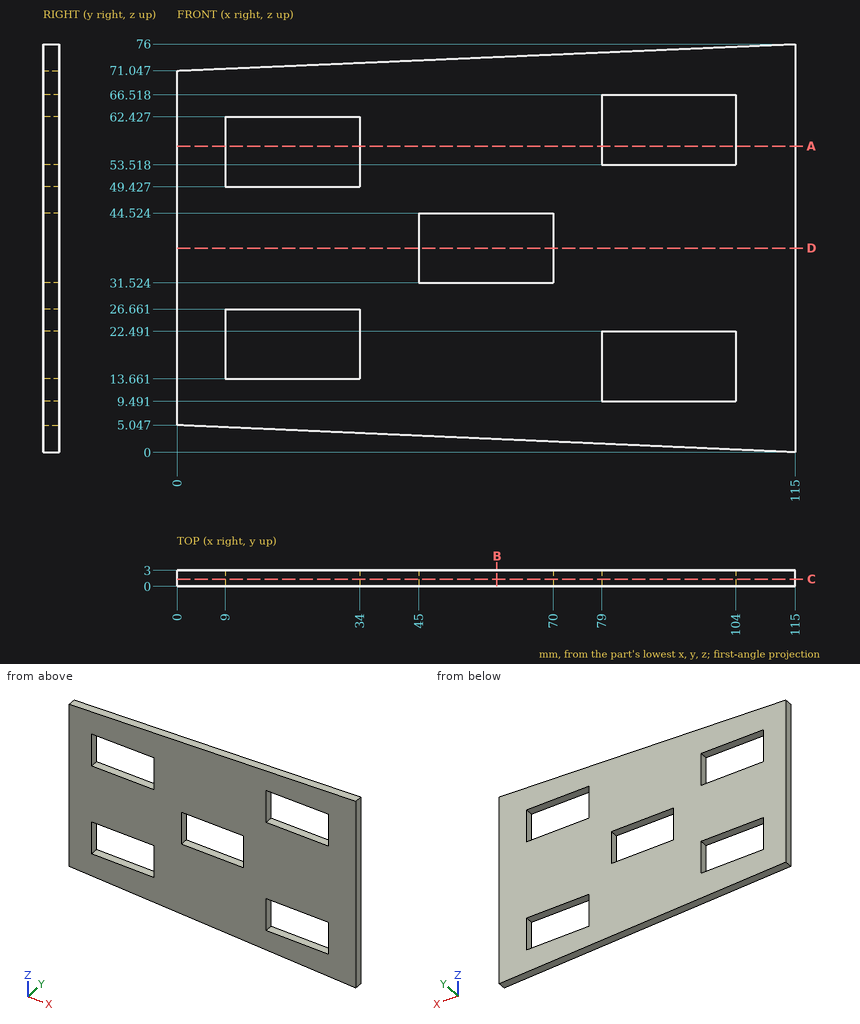
Design review of the part shown in the three views and the two pictorial views. Dimensions are in mm from the part's minimum x, y and z. Round coordinates to 2 decimals unless told otherwise and drop trailing zeros. Loops run counter-clockwise (first coordinate to the right, second up) from the corner with the lowest first, then second, coordinate; pieces in that order, holes last. Notation, with made-up numbers: (8, -11) -> (32, -11) arc R15 ccw to (32, 16) -> close; hole circle Ø4 at (-35.5, 51.25). An arc over 180 degrees is marked (long way). Return JSON: item names as keys, results as strings.
(1) Add section C-C on y = 1.35. Write out the cut boundary in (x, z), plus the area to 3 significant figures.
Solved:
{"outline": "(0, 5.05) -> (115, 0) -> (115, 76) -> (0, 71.05) -> close; hole (9, 13.66) -> (34, 13.66) -> (34, 26.66) -> (9, 26.66) -> close; hole (9, 49.43) -> (34, 49.43) -> (34, 62.43) -> (9, 62.43) -> close; hole (45, 31.52) -> (70, 31.52) -> (70, 44.52) -> (45, 44.52) -> close; hole (79, 9.49) -> (104, 9.49) -> (104, 22.49) -> (79, 22.49) -> close; hole (79, 53.52) -> (104, 53.52) -> (104, 66.52) -> (79, 66.52) -> close", "area": "6,540 mm2"}
(2) For pin 1 (0.9 mm diameter, centred on x = 18.5, y = 1, fed in from -Z); pin 2 (1 mm diameter, centred on x = 69.5, y = 0.5, fed in from +Z); pin 3 (0.9 mm diameter, centred on x = 63.5, y = 1.5, fed in from +Z), all flat-tipped, find the tip position at first contact; note any pin that passes through.
Solved:
{"pin 1": "z = 4.22", "pin 2": "z = 74.06", "pin 3": "z = 73.8"}
(3) Add section A-A on z = 57. Write out the cut boundary in (x, y), plus the area to 3 significant figures.
Solved:
{"outline": "(0, 0) -> (9, 0) -> (9, 3) -> (0, 3) -> close; (34, 0) -> (79, 0) -> (79, 3) -> (34, 3) -> close; (104, 0) -> (115, 0) -> (115, 3) -> (104, 3) -> close", "area": "195 mm2"}
(4) For line 1 (X direction, y = 2.6, z = 59); line 2 (X direction, y = 1.5, z = 33); line 3 (Z direction, x = 101, y = 1.55) (1 decimal), list the stretches that pass through material, from the lowest coordinate up.
Solved:
{"line 1": "0 to 9, 34 to 79, 104 to 115", "line 2": "0 to 45, 70 to 115", "line 3": "0.6 to 9.5, 22.5 to 53.5, 66.5 to 75.4"}
(5) Add section D-D on z = 38. Write out the cut boundary in (x, y), plus the area to 3 significant figures.
Solved:
{"outline": "(0, 0) -> (45, 0) -> (45, 3) -> (0, 3) -> close; (70, 0) -> (115, 0) -> (115, 3) -> (70, 3) -> close", "area": "270 mm2"}
(6) Add section B-B on x = 59.5. Write out the cut boundary in (y, z) (1 decimal).
Solved:
{"outline": "(0, 2.4) -> (3, 2.4) -> (3, 31.5) -> (0, 31.5) -> close; (0, 44.5) -> (3, 44.5) -> (3, 73.6) -> (0, 73.6) -> close"}
